Check sheet for the modelled part. Datum: model origin and axes. Units: mm. A direction names the side the tool comes from. Give positions to 0.01 mm unless a question says otherwise; leave off trailing zeros. Order: outer loops, then holes, each group sorted by start corner. A loop starts at its lowest first (then second) coordinate and runs counter-clockwise, first axis right, second up.
from build123d import *

# Parameters (mm, degrees)
F0_W     = 64
F0_H     = 56
F0_R     = 1.8
F0_R_2   = 4.5
F1_DEPTH = 8
F3_DEPTH = 30
F4_W     = 20
F4_H     = 24
F5_DEPTH = 25
F6_SIZE  = 4
F7_R     = 2


with BuildPart() as f1:
    # F0 (on Top) → F1 (new body)
    with BuildSketch(Plane.XY):
        Rectangle(F0_W, F0_H)
        with Locations((9.3431457505, -5.6568542495)):
            Circle(F0_R, mode=Mode.SUBTRACT)
        with Locations((20.6568542495, -5.6568542495)):
            Circle(F0_R, mode=Mode.SUBTRACT)
        with Locations((15, 0)):
            Circle(F0_R_2, mode=Mode.SUBTRACT)
        with Locations((9.3431457505, 5.6568542495)):
            Circle(F0_R, mode=Mode.SUBTRACT)
        with Locations((20.6568542495, 5.6568542495)):
            Circle(F0_R, mode=Mode.SUBTRACT)
    extrude(amount=F1_DEPTH)

    # F2 (on face) → F3 (cut)
    with BuildSketch(Plane(origin=(-32, 0, 0), x_dir=(0, -1, 0), z_dir=(-1, 0, 0))):
        with BuildLine():
            Line((-24.7241525946, 0), (-19.2758474054, 0))
            ThreePointArc((-19.2758474054, 0), (-22, 2.7241525946), (-24.7241525946, 0))
        make_face()
        with BuildLine():
            ThreePointArc((24.7241525946, 0), (22, 2.7241525946), (19.2758474054, 0))
            Line((19.2758474054, 0), (24.7241525946, 0))
        make_face()
    extrude(amount=-F3_DEPTH, mode=Mode.SUBTRACT)

    # F4 (on face) → F5 (cut)
    with BuildSketch(Plane.XY.offset(8)):
        with Locations((-22, 0)):
            Rectangle(F4_W, F4_H)
    extrude(amount=-F5_DEPTH, mode=Mode.SUBTRACT)

    # F6
    f6_edges = [f1.edges().sort_by_distance(p)[0] for p in [
        (-32, 12, 4),
        (-32, -12, 4),
    ]]
    chamfer(f6_edges, length=F6_SIZE)

    # F7
    f7_edges = [f1.edges().sort_by_distance(p)[0] for p in [
        (-12, 12, 4),
        (-12, -12, 4),
    ]]
    fillet(f7_edges, radius=F7_R)


solid = f1.part
1) Section check D-D, the plane x = -10.5. Record the cut outline in (y, z).
Recorded:
outline: (-28, 0) - (-24.72, 0) arc R2.72 cw to (-19.28, 0) - (19.28, 0) arc R2.72 cw to (24.72, 0) - (28, 0) - (28, 8) - (-28, 8) - close
2) Section check A-A, the plane x = -24.5. Record the cut outline in (y, z).
Recorded:
outline: (-28, 0) - (-24.72, 0) arc R2.72 cw to (-19.28, 0) - (-12, 0) - (-12, 8) - (-28, 8) - close; (12, 0) - (19.28, 0) arc R2.72 cw to (24.72, 0) - (28, 0) - (28, 8) - (12, 8) - close
3) Set-up check for faces 1 (the face through (-2, 22, 1)), 2 (the face through (-12.6, -11.43, 3.94)), 3 (the face through (10.504, 0.198, 3.944)): record each of +Z, -Z, +X, -X, +Y, -Y from which the full face is reachable in a straight line by a thin tool's end or side.
Recorded:
face 1: -Z, -X
face 2: +Z, -Z, -X
face 3: +Z, -Z
4) Section check B-B, the plane y = 0. Record the cut outline in (x, z).
Recorded:
outline: (-12, 0) - (10.5, 0) - (10.5, 8) - (-12, 8) - close; (19.5, 0) - (32, 0) - (32, 8) - (19.5, 8) - close
5) Material ranges on L1, parallel to Y at x = -25, z = 6; L2, parallel to Y at x = -26, z = 2; L3, parallel to X at y = -7, z = 4, recorded low to high.
Recorded:
L1: y = -28 to -12, 12 to 28
L2: y = -28 to -23.85, -20.15 to -12, 12 to 20.15, 23.85 to 28
L3: x = -12 to 8.14, 10.54 to 19.46, 21.86 to 32
6) Section check C-C, the plane z = 1.25. Record the cut outline in (x, y).
Recorded:
outline: (-32, -28) - (32, -28) - (32, 28) - (-32, 28) - (-32, 24.42) - (-2, 24.42) - (-2, 19.58) - (-32, 19.58) - (-32, 16) - (-28, 12) - (-14, 12) arc R2 cw to (-12, 10) - (-12, -10) arc R2 cw to (-14, -12) - (-28, -12) - (-32, -16) - (-32, -19.58) - (-2, -19.58) - (-2, -24.42) - (-32, -24.42) - close; hole circle Ø3.6 at (9.34, -5.66); hole circle Ø3.6 at (9.34, 5.66); hole circle Ø9 at (15, 0); hole circle Ø3.6 at (20.66, -5.66); hole circle Ø3.6 at (20.66, 5.66)
7) Depth check by flat-ended pin: pin 1 Ø1 at (x, y) = (22.5, 7) entering from -Z; pin 2 Ø3 at (x, y) = (9.34, -5.66) entering from -Z; pin 3 Ø1.4 at (y, z) = (-23.5, 1) entering from -X; pin 4 Ø1.5 at (y, z) = (-9, 6) entering from -X. Enter the tip coordinate at first touch or a pass-through.
Recorded:
pin 1: stops at z = 0
pin 2: passes through
pin 3: stops at x = -2
pin 4: stops at x = -12
